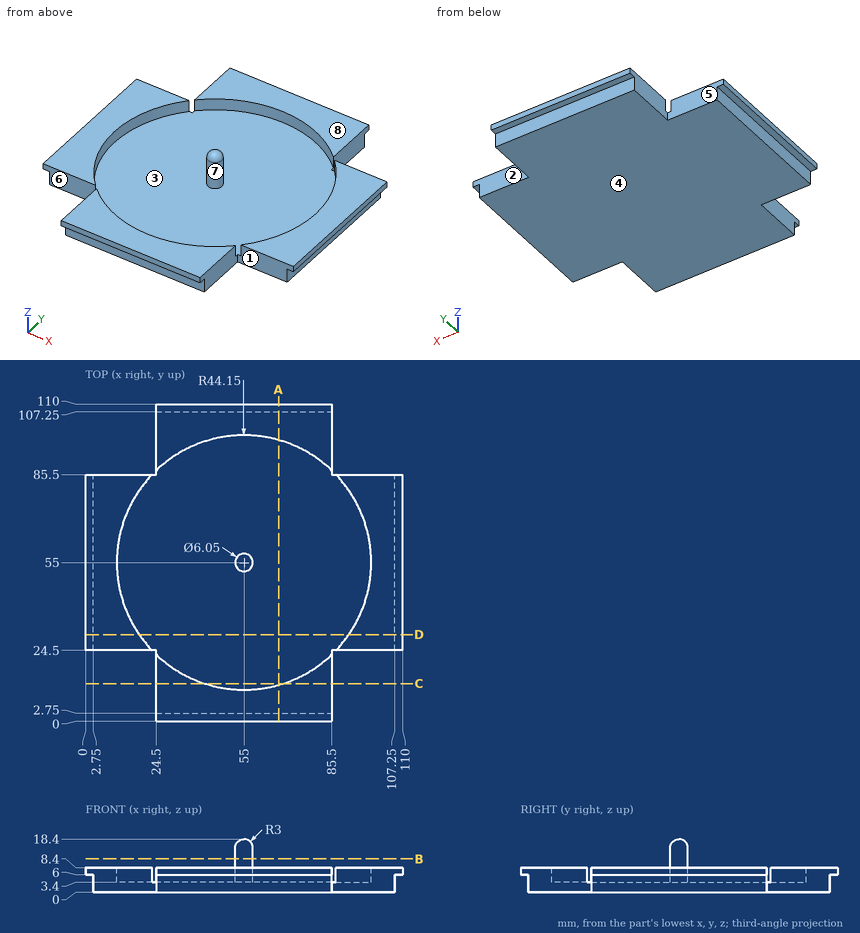
Input: dimensioned drawing with shaded views. Units: mm. Origin: part minimum x, y, z. A direction names the side the tool comes from. Coordinates: 2 decimals unless noted, no trailing zeros. Order: outer loops, then holes, each group sorted by start corner. A loop starts at its lowest first (then second) coordinate and runs counter-clockwise, first axis right, second up.
(1) Section query B-B (z = 11.5). Return the cut outline in (x, y) (3 decimals), plus the area to 3 significant figures.
(2) Access query for the marked faces 1, 2, 3 and 4. Directions: +Z, -Z, +X, -X, +Y, -Y. A direction counts if a zero-diameter tool reaches every point of the face in a straight line with its end or side. Return the directions, or none.
(3) Section query D-D (y = 30). Return the cut outline in (x, z), plus the area to 3 significant figures.
(4) First-contact query: pin 1 (6.5 mm diameter, centred on y = 9.5, z = 5, fed in from +X); pin 2 (4 mm diameter, centred on x = 12, z = 3, fed in from -Y); pin 3 (6 mm diameter, centred on y = 24.5, z = 11.5, fed in from +X); pin 4 (6.5 mm diameter, centred on y = 93, z = 2.5, fed in from -X). Flat tips, straight axial feed; report the tip coordinate or a pass-through.
(5) Draft query along Y for the marked faces 5, 6, 7 and 8. Return one class per face: pulls with the +Y half, pulls with the -Y half, needs draft (parallel to the pull), parting line crosses it, or undercut.
(6) Section query C-C (y = 13). Return the cut outline in (x, z), plus the area to 3 significant figures.
(7) Section query A-A (x = 67). Return the cut outline in (y, z).
(8) Material intervals for probe 1 along Z at (x, y) = (21.5, 52.5); probe 2 along X at (y, z) = (44, 2); probe 3 along X at (y, z) = (6, 6.5), sorted ascending.
Solution:
1. outline: circle Ø6.05 at (55, 55)
1. area: 28.7 mm2
2. face 1: +Z, -Z, +X, -Y
2. face 2: +Z, -Z, +X, +Y
2. face 3: +Z
2. face 4: -Z, +X, -X, +Y, -Y
3. outline: (0, 6) - (2.75, 6) - (2.75, 0) - (107.25, 0) - (107.25, 6) - (110, 6) - (110, 8.4) - (91.39, 8.4) - (91.39, 3.4) - (18.61, 3.4) - (18.61, 8.4) - (0, 8.4) - close
3. area: 527 mm2
4. pin 1: stops at x = 85.5
4. pin 2: stops at y = 24.5
4. pin 3: passes through
4. pin 4: stops at x = 24.5
5. face 5: pulls with the +Y half
5. face 6: pulls with the -Y half
5. face 7: undercut
5. face 8: needs draft
6. outline: (24.5, 0) - (85.5, 0) - (85.5, 8.4) - (68.61, 8.4) - (68.61, 3.4) - (41.39, 3.4) - (41.39, 8.4) - (24.5, 8.4) - close
6. area: 376 mm2
7. outline: (0, 6) - (2.75, 6) - (2.75, 0) - (107.25, 0) - (107.25, 6) - (110, 6) - (110, 8.4) - (97.49, 8.4) - (97.49, 3.4) - (12.51, 3.4) - (12.51, 8.4) - (0, 8.4) - close
8. probe 1: z = 0 to 3.4
8. probe 2: x = 2.75 to 107.25
8. probe 3: x = 24.5 to 85.5
